Can you work these out from the model? Positions are in its coordinate system, mm. A direction names the side the tool comes from. Round coordinates to 2 decimals unless told otherwise and drop trailing zeros. Loops run counter-clockwise (first coordinate to the right, second up) from the corner with the lowest first, then second, coordinate; pieces in that order, holes last. Notation, with made-up numbers: (27, 28) -> (49, 28) arc R30 cw to (49, 50) -> close; hole circle Ø3 at (-9.5, -27). An arc over 180 degrees is marked (long way). Write item = value, one per line.
Autodesk Inventor part; units mm, degrees
ref_plane "Work Plane1" through (12.5944, 0, 12.5944) normal (-0.7071, 0, 0.7071) x (0.7071, 0, 0.7071)
ref_plane "YZ Plane" through (0, 0, 0) normal (1, 0, 0) x (0, 1, 0)
ref_plane "XZ Plane" through (0, 0, 0) normal (0, 1, 0) x (-1, 0, 0)
sketch "Sketch1" plane through (0, 0, 0) normal (0, 1, 0) x (-1, 0, 0)
  line L0 (17.8112, 43) -> (43, 17.8112)
  line L1 (43, 17.8112) -> (43, -17.8112)
  line L2 (43, -17.8112) -> (17.8112, -43)
  line L3 (17.8112, -43) -> (-17.8112, -43)
  line L4 (-17.8112, -43) -> (-43, -17.8112)
  line L5 (-43, -17.8112) -> (-43, 17.8112)
  line L6 (-43, 17.8112) -> (-17.8112, 43)
  line L7 (-17.8112, 43) -> (17.8112, 43)
  point P0 (0, 0)
  point P1 (0, 0)
  point P2 (0, 43)
  dimension "d0" = 86
extrude "Extrusion1" add sketch "Sketch1" along normal blind 5
sketch "Sketch3" plane through (0, 0, 0) normal (0, -1, 0) x (1, 0, 0)
  line L0 (43, 17.8112) -> (43, -17.8112)
  line L1 (-15, 24) -> (-15, 26)
  line L2 (-15, 26) -> (0, 26)
  line L3 (0, 29) -> (-15, 29)
  line L4 (-15, 29) -> (-15, 31)
  line L5 (-15, 31) -> (0, 31)
  line L6 (0, 0) -> (0, 24) construction
  line L7 (0, 0) -> (-3.3479, 0) construction
  line L8 (0, 24) -> (-15, 24)
  line L9 (15, 24) -> (15, 26)
  line L10 (15, 26) -> (0, 26)
  line L11 (0, 29) -> (15, 29)
  line L12 (15, 29) -> (15, 31)
  line L13 (15, 31) -> (0, 31)
  line L14 (0, 24) -> (15, 24)
  line L15 (-15, -24) -> (-15, -26)
  line L16 (-15, -26) -> (0, -26)
  line L17 (0, -29) -> (-15, -29)
  line L18 (-15, -29) -> (-15, -31)
  line L19 (-15, -31) -> (0, -31)
  line L20 (0, -24) -> (-15, -24)
  line L21 (15, -24) -> (15, -26)
  line L22 (15, -26) -> (0, -26)
  line L23 (0, -29) -> (15, -29)
  line L24 (15, -29) -> (15, -31)
  line L25 (15, -31) -> (0, -31)
  line L26 (0, -24) -> (15, -24)
  line L27 (-17.8112, 43) -> (17.8112, 43)
  point P0 (11.5, 17.5)
  point P1 (-15, 25)
  point P2 (-7.5, 24)
  point P3 (15, 25)
  point P4 (7.5, 24)
  point P5 (11.5, -17.5)
  point P6 (-15, -25)
  point P7 (-7.5, -24)
  point P8 (15, -25)
  point P9 (7.5, -24)
  point P10 (0, 43)
  dimension "d21" = 2
  dimension "d22" = 3
  dimension "d23" = 2
  dimension "d25" = 15
  dimension "d30" = 12
extrude "Extrusion3" cut sketch "Sketch3" against normal blind 5
sketch "Sketch4" plane through (0, 5, 0) normal (0, 1, 0) x (1, 0, 0)
  circle A0 centre (0, 0) radius 4.4721
extrude "Extrusion4" cut sketch "Sketch4" against normal blind 0.01
ref_plane "Work Plane1" through (12.5944, 0, 12.5944) normal (-0.7071, 0, 0.7071) x (0.7071, 0, 0.7071)
sketch "Sketch5" plane through (12.5944, 0, 12.5944) normal (-0.7071, 0, 0.7071) x (0.7071, 0, 0.7071)
  line L0 (25.1888, 5) -> (19.1888, 5)
  line L1 (25.1888, 5) -> (0, 5)
  line L2 (19.1888, 5) -> (19.1888, 9) construction
  line L3 (19.1888, 9) -> (23.1888, 9) construction
  circle A0 centre (23.1888, 9) radius 3
  circle A1 centre (23.1888, 9) radius 1.6
  line L4 (25.1888, 5) -> (26.0788, 8.195)
  line L5 (15.1888, 5) -> (21.0249, 11.0778)
  line L6 (15.1888, 5) -> (19.1888, 5)
  line L7 (19.1888, 9.1657) -> (18.1888, 5)
  point P0 (-17.8112, 0)
  point P1 (-17.8112, 0)
  point P2 (-107.2923, -20.1826)
  point P3 (-107.2923, -23.1826)
  point P4 (15.1888, 5)
  dimension "d33" = 6
  dimension "d34" = 4
  dimension "d35" = 4
  dimension "d36" = 6
  dimension "d37" = 3.2
  dimension "d38" = 10
  dimension "d39" = 1
extrude "Extrusion5" add sketch "Sketch5" along normal mid plane 5.5
pattern_circular "Circular Pattern2" count 4 over 360 about axis through (0, 5, 0) along (0, -1, 0) of "Extrusion5"
sketch "Sketch6" plane through (0, 5, 0) normal (0, 1, 0) x (1, 0, 0)
  line L0 (0, 0) -> (30.1227, 30.1227) construction
  line L1 (32.0673, 28.1782) -> (28.1782, 32.0673) construction
  line L2 (-15.05, -15.05) -> (15.05, -15.05) construction
  line L3 (15.05, -15.05) -> (15.05, 15.05) construction
  line L4 (15.05, 15.05) -> (-15.05, 15.05) construction
  line L5 (-15.05, 15.05) -> (-15.05, -15.05) construction
  line L6 (-15.05, -15.05) -> (15.05, 15.05) construction
  line L7 (15.05, -15.05) -> (-15.05, 15.05) construction
  dimension "d45" = 30.1
  dimension "d46" = 30.1
hole "Hole1" at (-15.05, 5, -15.05) at (-15.05, 5, 15.05) at (15.05, 5, -15.05) at (15.05, 5, 15.05) direction (0, -1, 0) diameter 4.2 end through all
sketch "Sketch7" plane through (0, 5, 0) normal (0, 1, 0) x (1, 0, 0)
  line L0 (-18, -18) -> (18, -18) construction
  line L1 (18, -18) -> (18, 18) construction
  line L2 (18, 18) -> (-18, 18) construction
  line L3 (-18, 18) -> (-18, -18) construction
  line L4 (-18, -18) -> (18, 18) construction
  line L5 (18, -18) -> (-18, 18) construction
  line L6 (-19, -29) -> (19, -29) construction
  line L7 (19, -29) -> (19, 29) construction
  line L8 (19, 29) -> (-19, 29) construction
  line L9 (-19, 29) -> (-19, -29) construction
  circle A0 centre (0, 0) radius 4.4721 construction
  line L10 (-19, -29) -> (19, 29) construction
  line L11 (19, -29) -> (-19, 29) construction
  dimension "d59" = 36
  dimension "d60" = 36
  dimension "d61" = 58
  dimension "d62" = 38
hole "Hole2" at (-19, 5, -29) at (19, 5, -29) at (19, 5, 29) at (-19, 5, 29) direction (0, -1, 0) diameter 3.2 end through all
properties part number "bottom"
1. We'd pull the mould along X, two halves only. Please class faces 1 (the flat face through (-30.58, 2.46, -30.23)), 2 (the cylindrical face through (-16.82, 2.46, 16.18)), 3 (the flat face through (0, 2, 43)): released by +X, released by -X, zero draft, split by the parting line, or undercut.
Entries:
face_1 = released by -X
face_2 = undercut
face_3 = zero draft
2. I'm going to push flat-ended pins straight in: pin 1 (2 mm diameter, centred on x = 34.5, y = 2, fed in from -Z); pin 2 (3.5 mm diameter, centred on x = -19, z = 29, fed in from -Y); pin 3 (5 mm diameter, centred on y = 4.5, z = -28.5, fed in from +X); pin 4 (1 mm diameter, centred on y = 1.5, z = -25, fed in from -X). Where does each tip first touch, or does it pass through?
Entries:
pin_1 = -27.31
pin_2 = 0
pin_3 = 34.81
pin_4 = -36.31
3. Suppose I cut it at B-B, the plane x = 0. Count the separate pieces of the cut face and the enclosed holes in it, and give its area (3 significant figures).
Entries:
separate_pieces = 5
enclosed_holes = 0
area = 390 mm²
4. Suppose I cut it at A-A, the plane z = -15.05. List the corners of the cut face in (x, y) for me, and give its area (3 significant figures).
Entries:
outline = (-43, 0) -> (-17.15, 0) -> (-17.15, 5) -> (-43, 5) -> close; (-12.95, 0) -> (12.95, 0) -> (12.95, 5) -> (-12.95, 5) -> close; (17.15, 0) -> (43, 0) -> (43, 5) -> (17.15, 5) -> close
area = 388 mm²
5. I need wall thicknesses on line 1 (Z direction, x = 15.05, y = 3.25); line 2 (Z direction, x = 1, y = 0.5). Which ranges of each line are inside material? Lowest first, please. Write a range as [from, to].
Entries:
line_1 = [-43, -17.15], [-12.95, 12.95], [17.15, 43]
line_2 = [-43, -31], [-29, -26], [-24, 24], [26, 29], [31, 43]
6. For faces 4 (the flat face through (15, 2, 25)), 5 (the flat face through (-26.09, 7.77, 29.98)), 6 (the flat face through (25.34, 8, -25.4)), 7 (the flat face through (29.98, 7.77, 26.09)), which set-ups out of +Z, -Z, +X, -X, +Y, -Y let a thin tool reach every point of the face, with its end or its side?
Entries:
face_4 = +Y, -Y
face_5 = +Z, +Y
face_6 = +Y
face_7 = +X, +Y
